from build123d import *

# Parameters (mm, degrees)
F0_W     = 465
F0_H     = 18
F0_W_2   = 457
F0_H_2   = 10
F0_H_3   = 6
F1_DEPTH = 20
F2_START = 10
F2_DEPTH = 10


with BuildPart() as f1:
    # F0 (on Top) → F1 (new body)
    with BuildSketch(Plane.XY):
        with Locations((252.0387396961, -41.0362935066)):
            Rectangle(F0_W, F0_H)
        with Locations((252.0387396961, -41.0362935066)):
            Rectangle(F0_W_2, F0_H_2, mode=Mode.SUBTRACT)
        with Locations((252.0387396961, -53.0362935066)):
            Rectangle(F0_W, F0_H_3)
    extrude(amount=F1_DEPTH)

    # F0 (on Top) → F2 (join)
    with BuildSketch(Plane.XY.offset(F2_START)):
        with Locations((252.0387396961, -41.0362935066)):
            Rectangle(F0_W_2, F0_H_2)
    extrude(amount=F2_DEPTH)


solid = f1.part
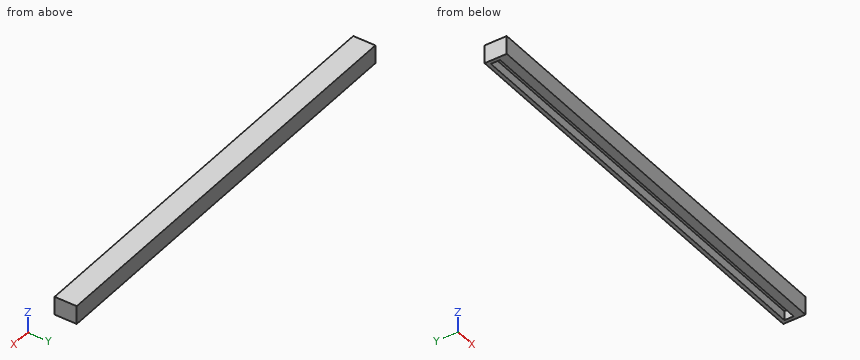
Here's how the part is built. I have some questions about the finished solid (model axes, mm). Round coordinates to 2 decimals unless told otherwise and drop trailing zeros. Order: outer loops, then holes, each group sorted by start corner. A loop starts at its lowest first (then second) coordinate and runs counter-clockwise, first axis right, second up. Notation, with made-up numbers: (-8.75, 43.5) -> (37.25, 43.5) arc R8 ccw to (37.25, 49.5) -> close; hole circle Ø10 at (41, -20.75). An arc over 180 degrees is marked (long way). Return JSON: item names as keys, results as strings.
Q1. I need wall thicknesses on line 1 along X through (y, z) = (-37, 2.75); line 2 along Y through (x, z) = (186.5, 5); line 3 along Z through (x, y) = (444, -44.75). Which ranges of each line are inside material? Lowest first, please. Write a range as from..to.
Filled sheet:
{"line 1": "x = 19.54..23.54, 480.54..484.54", "line 2": "y = -56.04..-46.04, -36.04..-32.04", "line 3": "z = 10..20"}
Q2. If we section it at A-A on z = 5.25: List the corners of the cut face in (x, y) for me, plus the area to 3 significant figures.
Filled sheet:
{"outline": "(19.54, -56.04) -> (484.54, -56.04) -> (484.54, -32.04) -> (19.54, -32.04) -> close; hole (23.54, -46.04) -> (480.54, -46.04) -> (480.54, -36.04) -> (23.54, -36.04) -> close", "area": "6,590 mm^2"}
Q3. For pin 1 Ø11 at (x, y) = (192, -39.5) entering from -Z, with a flat end and sliding along its axis, tell me the tip position at first contact or that it passes through.
Filled sheet:
{"pin 1": "stops at z = 0"}
Q4. If we section it at B-B on y = -41: List the corners of the cut face in (x, z) for me.
Filled sheet:
{"outline": "(19.54, 0) -> (23.54, 0) -> (23.54, 10) -> (480.54, 10) -> (480.54, 0) -> (484.54, 0) -> (484.54, 20) -> (19.54, 20) -> close"}
Q5. If we section it at C-C on x = 49: List the corners of the cut face in (y, z) for me.
Filled sheet:
{"outline": "(-56.04, 0) -> (-46.04, 0) -> (-46.04, 10) -> (-36.04, 10) -> (-36.04, 0) -> (-32.04, 0) -> (-32.04, 20) -> (-56.04, 20) -> close"}
